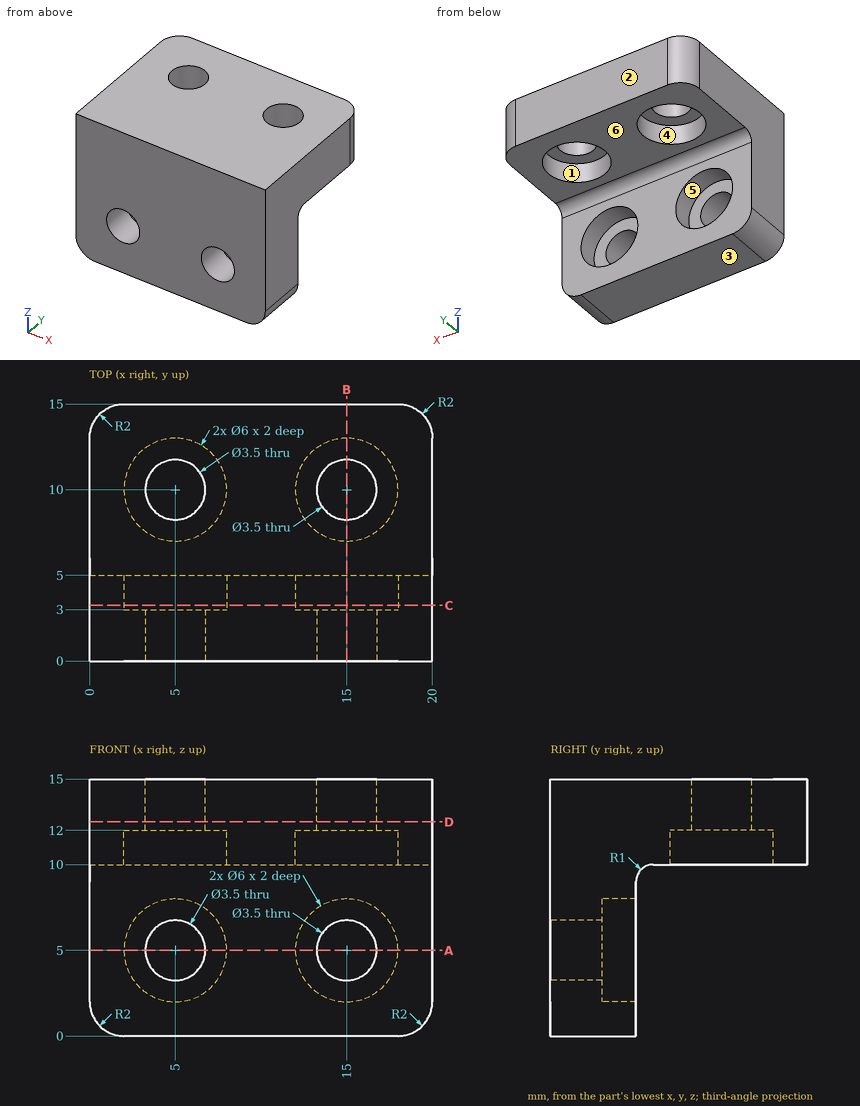
Here's the drawing with two shaded views (mm, measured from the low corner). I have some questions. A direction names the side the tool comes from. Round coordinates to 2 decimals unless told otherwise and drop trailing zeros. Loops run counter-clockwise (first coordinate to the right, second up) from the corner with the lowest first, then second, coordinate; pieces in that order, holes last.
1. Suppose I cut it at C-C, the plane y = 3.25. Please give me the cut outline in (x, z), and give its area (3 significant figures).
Answers:
outline: (0, 2) arc R2 ccw to (2, 0) - (18, 0) arc R2 ccw to (20, 2) - (20, 15) - (0, 15) - close; hole circle Ø6 at (5, 5); hole circle Ø6 at (15, 5)
area: 242 mm2
2. Suppose I cut it at B-B, the plane x = 15. Please give me the cut outline in (y, z), and give its area (3 significant figures).
Answers:
outline: (0, 0) - (5, 0) - (5, 2) - (3, 2) - (3, 3.25) - (0, 3.25) - close; (0, 6.75) - (3, 6.75) - (3, 8) - (5, 8) - (5, 9) arc R1 cw to (6, 10) - (7, 10) - (7, 12) - (8.25, 12) - (8.25, 15) - (0, 15) - close; (11.75, 12) - (13, 12) - (13, 10) - (15, 10) - (15, 15) - (11.75, 15) - close
area: 80.2 mm2
3. For the marked faces 4, 5 and 6, which set-ups out of +Z, -Z, +X, -X, +Y, -Y let a thin tool reach every point of the face, with its end or its side?
Answers:
face 4: -Z
face 5: +Y
face 6: -Z, +X, -X, +Y
4. Will these pins go through, and if not, where does the flat tip stop? pin 1 (5.5 mm diameter, centred on x = 5, y = 10, fed in from -Z); pin 2 (3 mm diameter, centred on x = 5, z = 5, fed in from +Y); pin 3 (6.5 mm diameter, centred on x = 14, y = 9, fed in from -Z); pin 4 (2.5 mm diameter, centred on x = 8, z = 6, fed in from +Y).
Answers:
pin 1: stops at z = 12
pin 2: passes through
pin 3: stops at z = 9.97
pin 4: stops at y = 5
5. Suppose I cut it at D-D, the plane z = 12.5. Please give me the cut outline in (x, y).
Answers:
outline: (0, 0) - (20, 0) - (20, 13) arc R2 ccw to (18, 15) - (2, 15) arc R2 ccw to (0, 13) - close; hole circle Ø3.5 at (5, 10); hole circle Ø3.5 at (15, 10)
6. Suppose I cut it at A-A, the plane z = 5. Please give me the cut outline in (x, y), and give its area (3 significant figures).
Answers:
outline: (0, 0) - (3.25, 0) - (3.25, 3) - (2, 3) - (2, 5) - (0, 5) - close; (6.75, 0) - (13.25, 0) - (13.25, 3) - (12, 3) - (12, 5) - (8, 5) - (8, 3) - (6.75, 3) - close; (16.75, 0) - (20, 0) - (20, 5) - (18, 5) - (18, 3) - (16.75, 3) - close
area: 55.0 mm2
7. If I drill on probe 1 along X at (y, z) = (1.2, 5); probe 2 along X at (y, z) = (3.85, 5); probe 3 along Y at (x, z) = (5, 10.8), over which ranges is the centre line in solid material (lowest first)?
Answers:
probe 1: x = 0 to 3.25, 6.75 to 13.25, 16.75 to 20
probe 2: x = 0 to 2, 8 to 12, 18 to 20
probe 3: y = 0 to 7, 13 to 15
8. Thinking about a two-plate mould opening in Y: for the marked faces 1, 2 and 3, which applies, released by +Y, released by -Y, zero draft, split by the parting line, or undercut?
Answers:
face 1: undercut
face 2: released by +Y
face 3: zero draft
